The model under review builds one solid part; all positions refer to its coordinate system, in mm. A direction names the side the tool comes from. Round coordinates to 2 decimals unless told otherwise and drop trailing zeros. Write each loop counter-clockwise with the first axis right and the second up, starting at its lowest first coordinate (ties: lowest second). Pieces come first, ordered by that corner, then holes. Notation, with made-up numbers: (-4, -31) -> (48, -31) arc R32 ccw to (48, -2) -> close; hole circle Ø2 at (21.25, -34). An arc over 180 degrees is marked (long way). Answer as a JSON object with one key per item and string values. Group by question number.
1) We need section C-C, the plane x = -4.5. Write out the cut boundary in (y, z), then the cut area to 3 significant figures.
2) Insertion check: pin 1 Ø1 at (y, z) = (1.5, 21.5) entering from +X; pin 2 Ø1.5 at (x, y) = (12, 1) entering from -Z; pin 3 Ø1.7 at (x, z) = (13, 7) entering from -Y; pin 4 Ø14.5 at (x, z) = (0, 0) entering from -Y. Each pin has a flat end and moves straight along its axis. Give the tip position at first contact, or say it passes through.
3) We need section B-B, the plane z = 72.5. Write out the cut boundary in (x, y), then the cut area to 3 significant figures.
4) We need section D-D, the plane z = 6.75. Write out the cut boundary in (x, y).
5) We need section A-A, the plane x = 0. Write out the cut boundary in (y, z), then the cut area to 3 significant figures.
6) Mouldability with a two-part tool opening along Z and no side actions: class faces 1 (the flat face through (-13.73, 0.06, 37.17)), 2 (the cylindrical face through (10.46, 1.54, 7.69)) as pulls with the +Z half, pulls with the -Z half, needs draft (parallel to the pull), parting line crosses it, or undercut.
7) To check wall thickness, follow probe 1 along Z at (x, y) = (0, -2.65); probe 2 along Z at (x, y) = (0, 2.2); probe 3 along Z at (x, y) = (3.5, 1.5). State the ranges of each line that lie inside material, in increasing order. Write a range as [from, to].
8) Machinability: for faces 3 (the flat face through (-7.65, 0.06, 47.46)), 4 (the cylindrical face through (10.399, -2.521, 9.234)), which of the approach directions +Z, -Z, +X, -X, +Y, -Y give a long, thin tool a straight path to every point of the face, cutting with its end or side? Answer none if there is none.
from build123d import *

# Parameters (mm, degrees)
EXTRUDE_1_DEPTH                = 8
CUT_EXTRUDE_1_DEPTH            = 9
CUT_EXTRUDE_2_DEPTH            = 9
CUT_EXTRUDE_3_DEPTH            = 9
CUT_EXTRUDE_4_DEPTH            = 9
CUT_EXTRUDE_5_DEPTH            = 9
CUT_EXTRUDE_6_DEPTH            = 9
HOLE_WIZARD_16_0_16_1_D        = 16.1
HOLE_WIZARD_16_0_16_1_DEPTH    = 8
HOLE_WIZARD_13_0_13_1_D        = 13.1
HOLE_WIZARD_13_0_13_1_DEPTH    = 8
HOLE_WIZARD_M2_5_1_D           = 3.1
HOLE_WIZARD_M2_5_1_DEPTH       = 8
HOLE_WIZARD_M2_5_1_CBORE_D     = 5.6
HOLE_WIZARD_M2_5_1_CBORE_DEPTH = 3
FILLET_1_R                     = 0.5


with BuildPart() as part:
    # 草图1 → 凸台-拉伸1 (new body)
    with BuildSketch(Plane(origin=(0, 4, 0), x_dir=(1, 0, 0), z_dir=(0, 1, 0))):
        with BuildLine():
            Line((-17.406109606, -1.810344828), (-9.946348346, -73.534482759))
            ThreePointArc((-9.946348346, -73.534482759), (0, -82.5), (9.946348346, -73.534482759))
            Line((9.946348346, -73.534482759), (17.406109606, -1.810344828))
            ThreePointArc((17.406109606, -1.810344828), (0, 17.5), (-17.406109606, -1.810344828))
        make_face()
    extrude(amount=-EXTRUDE_1_DEPTH)

    # 草图2 → 切除-拉伸1 (cut, through all)
    with BuildSketch(Plane(origin=(0, 4, 0), x_dir=(-1, 0, 0), z_dir=(0, 1, 0))):
        with BuildLine():
            Line((2, 43.750482659), (2, 41))
            Line((2, 41), (6.923179382, 36.483241979))
            ThreePointArc((6.923179382, 36.483241979), (7.485869271, 36.40499598), (7.758515386, 36.903399876))
            Line((7.758515386, 36.903399876), (7.518784371, 39.208366459))
            Line((7.518784371, 39.208366459), (2.861977096, 44.095406683))
            ThreePointArc((2.861977096, 44.095406683), (2.314242831, 44.214696268), (2, 43.750482659))
        make_face()
    extrude(amount=-CUT_EXTRUDE_1_DEPTH, mode=Mode.SUBTRACT)

    # 草图3 → 切除-拉伸2 (cut, through all)
    with BuildSketch(Plane(origin=(0, 4, 0), x_dir=(-1, 0, 0), z_dir=(0, 1, 0))):
        with BuildLine():
            Line((-6.923179382, 36.483241979), (-2, 41))
            Line((-2, 41), (-2, 43.750482659))
            ThreePointArc((-2, 43.750482659), (-2.314242831, 44.214696268), (-2.861977096, 44.095406683))
            Line((-2.861977096, 44.095406683), (-7.518784371, 39.208366459))
            Line((-7.518784371, 39.208366459), (-7.758515386, 36.903399876))
            ThreePointArc((-7.758515386, 36.903399876), (-7.485869271, 36.40499598), (-6.923179382, 36.483241979))
        make_face()
    extrude(amount=-CUT_EXTRUDE_2_DEPTH, mode=Mode.SUBTRACT)

    # 草图4 → 切除-拉伸3 (cut, through all)
    with BuildSketch(Plane(origin=(0, 4, 0), x_dir=(-1, 0, 0), z_dir=(0, 1, 0))):
        with BuildLine():
            Line((2, 53.250482659), (2, 50.5))
            Line((2, 50.5), (6.923179382, 45.983241979))
            ThreePointArc((6.923179382, 45.983241979), (7.485869271, 45.90499598), (7.758515386, 46.403399876))
            Line((7.758515386, 46.403399876), (7.518784371, 48.708366459))
            Line((7.518784371, 48.708366459), (2.861977096, 53.595406683))
            ThreePointArc((2.861977096, 53.595406683), (2.314242831, 53.714696268), (2, 53.250482659))
        make_face()
    extrude(amount=-CUT_EXTRUDE_3_DEPTH, mode=Mode.SUBTRACT)

    # 草图5 → 切除-拉伸4 (cut, through all)
    with BuildSketch(Plane(origin=(0, 4, 0), x_dir=(-1, 0, 0), z_dir=(0, 1, 0))):
        with BuildLine():
            Line((-6.923179382, 45.983241979), (-2, 50.5))
            Line((-2, 50.5), (-2, 53.250482659))
            ThreePointArc((-2, 53.250482659), (-2.314242831, 53.714696268), (-2.861977096, 53.595406683))
            Line((-2.861977096, 53.595406683), (-7.518784371, 48.708366459))
            Line((-7.518784371, 48.708366459), (-7.758515386, 46.403399876))
            ThreePointArc((-7.758515386, 46.403399876), (-7.485869271, 45.90499598), (-6.923179382, 45.983241979))
        make_face()
    extrude(amount=-CUT_EXTRUDE_4_DEPTH, mode=Mode.SUBTRACT)

    # 草图6 → 切除-拉伸5 (cut, through all)
    with BuildSketch(Plane(origin=(0, 4, 0), x_dir=(-1, 0, 0), z_dir=(0, 1, 0))):
        with BuildLine():
            Line((2, 62.750482659), (2, 60))
            Line((2, 60), (6.923179382, 55.483241979))
            ThreePointArc((6.923179382, 55.483241979), (7.485869271, 55.40499598), (7.758515386, 55.903399876))
            Line((7.758515386, 55.903399876), (7.518784371, 58.208366459))
            Line((7.518784371, 58.208366459), (2.861977096, 63.095406683))
            ThreePointArc((2.861977096, 63.095406683), (2.314242831, 63.214696268), (2, 62.750482659))
        make_face()
    extrude(amount=-CUT_EXTRUDE_5_DEPTH, mode=Mode.SUBTRACT)

    # 草图7 → 切除-拉伸6 (cut, through all)
    with BuildSketch(Plane.XZ.offset(4)):
        with BuildLine():
            Line((2, 62.750482659), (2, 60))
            Line((2, 60), (6.923179382, 55.483241979))
            ThreePointArc((6.923179382, 55.483241979), (7.485869271, 55.40499598), (7.758515386, 55.903399876))
            Line((7.758515386, 55.903399876), (7.518784371, 58.208366459))
            Line((7.518784371, 58.208366459), (2.861977096, 63.095406683))
            ThreePointArc((2.861977096, 63.095406683), (2.314242831, 63.214696268), (2, 62.750482659))
        make_face()
    extrude(amount=-CUT_EXTRUDE_6_DEPTH, mode=Mode.SUBTRACT)

    # Ø16.0 (16) 直径孔1
    with Locations(Plane(origin=(0, -4, 0), x_dir=(-1, 0, 0), z_dir=(0, -1, 0))):
        with Locations((0, 0)):
            Hole(HOLE_WIZARD_16_0_16_1_D / 2, depth=HOLE_WIZARD_16_0_16_1_DEPTH)

    # Ø13.0 (13) 直径孔1
    with Locations(Plane(origin=(0, 4, 0), x_dir=(1, 0, 0), z_dir=(0, 1, 0))):
        with Locations((0, -72.5)):
            Hole(HOLE_WIZARD_13_0_13_1_D / 2, depth=HOLE_WIZARD_13_0_13_1_DEPTH)

    # M2.5 六角头机械螺钉的柱形沉头孔1
    with Locations(Plane(origin=(0, -4, 0), x_dir=(-1, 0, 0), z_dir=(0, -1, 0))):
        with Locations((11.691342951, -6.75), (11.691342951, 6.75), (0, 13.5), (-11.691342951, 6.75), (-11.691342951, -6.75), (0, -13.5)):
            CounterBoreHole(HOLE_WIZARD_M2_5_1_D / 2, HOLE_WIZARD_M2_5_1_CBORE_D / 2, HOLE_WIZARD_M2_5_1_CBORE_DEPTH, depth=HOLE_WIZARD_M2_5_1_DEPTH)

    # 圆角1
    fillet_1_edges = [part.edges().sort_by_distance(p)[0] for p in [
        (-7.518784371, 0, 58.208366459),
        (-2, 0, 60),
        (7.518784371, 0, 58.208366459),
        (2, 0, 60),
        (-7.518784371, 0, 39.208366459),
        (-2, 0, 41),
        (7.518784371, 0, 39.208366459),
        (2, 0, 41),
        (-7.518784371, 0, 48.708366459),
        (-2, 0, 50.5),
        (7.518784371, 0, 48.708366459),
        (2, 0, 50.5),
    ]]
    fillet(fillet_1_edges, radius=FILLET_1_R)


solid = part.part
Here are the results:
{
 "1": {"outline": "(-4, -16.91) -> (4, -16.91) -> (4, -6.67) -> (-4, -6.67) -> close; (-4, 6.67) -> (4, 6.67) -> (4, 38.71) -> (-4, 38.71) -> close; (-4, 42.38) -> (4, 42.38) -> (4, 48.21) -> (-4, 48.21) -> close; (-4, 51.88) -> (4, 51.88) -> (4, 57.71) -> (-4, 57.71) -> close; (-4, 61.38) -> (4, 61.38) -> (4, 67.74) -> (-4, 67.74) -> close; (-4, 77.26) -> (4, 77.26) -> (4, 81.43) -> (-4, 81.43) -> close", "area": "516 mm^2"},
 "2": {"pin 1": "stops at x = 15.41", "pin 2": "stops at z = -13.4", "pin 3": "stops at y = -1", "pin 4": "passes through"},
 "3": {"outline": "(-10.05, -4) -> (-6.55, -4) -> (-6.55, 4) -> (-10.05, 4) -> close; (6.55, -4) -> (10.05, -4) -> (10.05, 4) -> (6.55, 4) -> close", "area": "56.1 mm^2"},
 "4": {"outline": "(-16.89, -4) -> (-14.49, -4) -> (-14.49, -1) -> (-13.24, -1) -> (-13.24, 4) -> (-16.89, 4) -> close; (-10.14, -1) -> (-8.89, -1) -> (-8.89, -4) -> (-4.39, -4) -> (-4.39, 4) -> (-10.14, 4) -> close; (4.39, -4) -> (8.89, -4) -> (8.89, -1) -> (10.14, -1) -> (10.14, 4) -> (4.39, 4) -> close; (13.24, -1) -> (14.49, -1) -> (14.49, -4) -> (16.89, -4) -> (16.89, 4) -> (13.24, 4) -> close"},
 "5": {"outline": "(-4, -17.5) -> (4, -17.5) -> (4, -15.05) -> (-1, -15.05) -> (-1, -16.3) -> (-4, -16.3) -> close; (-4, -10.7) -> (-1, -10.7) -> (-1, -11.95) -> (4, -11.95) -> (4, -8.05) -> (-4, -8.05) -> close; (-4, 8.05) -> (4, 8.05) -> (4, 11.95) -> (-1, 11.95) -> (-1, 10.7) -> (-4, 10.7) -> close; (-4, 16.3) -> (-1, 16.3) -> (-1, 15.05) -> (4, 15.05) -> (4, 65.95) -> (-4, 65.95) -> close; (-4, 79.05) -> (4, 79.05) -> (4, 82.5) -> (-4, 82.5) -> close", "area": "502 mm^2"},
 "6": {"face 1": "pulls with the +Z half", "face 2": "undercut"},
 "7": {"probe 1": "z = [-17.5, -16.3], [-10.7, -8.05], [8.05, 10.7], [16.3, 65.95], [79.05, 82.5]", "probe 2": "z = [-17.5, -15.05], [-11.95, -8.05], [8.05, 11.95], [15.05, 65.95], [79.05, 82.5]", "probe 3": "z = [-17.15, -7.25], [7.25, 39.62], [43.43, 49.12], [52.93, 58.62], [62.43, 66.96], [78.04, 81.87]"},
 "8": {"face 3": "+Y, -Y", "face 4": "-Y"}
}
